Geometry check sheet. Reference: the model listing, model coordinates, mm. A direction names the side the tool comes from. Give positions to 0.01 mm unless a question says otherwise; leave off trailing zeros. Order: outer loops, then holes, each group sorted by start corner. A loop starts at its lowest first (then second) coordinate and runs counter-clockwise, first axis right, second up. Notation, with made-up numbers: (64.25, 38) - (114.25, 38) arc R27 cw to (114.25, 73) - close; hole circle Ø5 at (-28.75, 57.5). An arc over 180 degrees is marked (long way). Put each result on its own line as item: value. Start each with the question number.
```python
from build123d import *

# Parameters (mm, degrees)
CROQUIS3_W     = 1.65
CROQUIS3_H     = 8.851
MATRIZC1_COUNT = 2
MATRIZC1_ANGLE = 90


with BuildPart() as part:
    # Croquis1 → Revolución1 (revolve)
    with BuildSketch(Plane.XY):
        Polygon((8.85, 6.45), (8.85, 0), (2.5, 0), (2.5, 20.75), (8.85, 20.75), (8.85, 19.35), (6, 19.35), (6, 6.45), align=None)
    revolve(axis=Axis((0, 0, 0), (0, 1, 0)))

    # Croquis3 → Taladro roscado M41 (revolve, cut)
    with BuildSketch(Plane(origin=(0, 3.225, 0), x_dir=(0, 1, 0), z_dir=(1, 0, 0))):
        with Locations((0.825, 4.4255)):
            Rectangle(CROQUIS3_W, CROQUIS3_H)
    taladro_roscado_m41 = revolve(axis=Axis((0, 3.225, -6.35), (0, 0, 1)), mode=Mode.SUBTRACT)

    # MatrizC1: Taladro roscado M41 ×2 about axis
    matrizc1_axis = Axis((0, 0, 0), (0, -1, 0))
    for i in range(1, MATRIZC1_COUNT):
        add(taladro_roscado_m41.rotate(matrizc1_axis, i * MATRIZC1_ANGLE / (MATRIZC1_COUNT - 1)), mode=Mode.SUBTRACT)


solid = part.part
```
Item 1: Cross-section at A-A (z = 0). Enter the section's corners in (x, y) (3 decimals).
Item 2: Release check for a two-part mould opening along Y. For faces 1 (the face through (-0.073, 1.577, 5.415)), 2 (the face through (8.44, 20.04, -2.66)), 3 (the face through (2, 0, 2)), 4 (the face through (6, 19.35, 2)) record: +Y half, -Y half, draft (parallel to the pull), parting line (faces both ways), or undercut.
Item 3: Cross-section at C-C (z = 7.75). Enter the section's corners in (x, y) (3 decimals).
Item 4: Thickness scan on line 1 along Z through (x, y) = (0, 10.5); line 2 along Y through (x, z) = (-5.5, 5.75). Record the ranges inside material, lowest first.
Item 5: Cross-section at B-B (x = -7.5). Enter the section's corners in (y, z) (3 decimals), and give its area (3 significant figures).
Item 6: Cross-section at D-D (y = 2). Enter the section's corners in (x, z), and give its area (3 significant figures).
Item 7: Set-up check for faces 5 (the face through (8.44, 3.18, -2.66)), 6 (the face through (-5.413, 1.577, -0.073)), 7 (the face through (-6, 13, 0)): record each of +Z, -Z, +X, -X, +Y, -Y from which the full face is reachable in a straight line by a thin tool's end or side.
Item 8: Gauge pin test, flat ends, axial feed: pin 1 Ø10 at (y, z) = (14.5, 3) entering from -X; pin 2 Ø1.5 at (y, z) = (13, -2.5) entering from +X; pin 3 Ø2.5 at (y, z) = (3.225, 0) entering from -X; pin 4 Ø9 at (x, z) = (-2.5, -2.5) entering from -Y. Record the tip position at first contact, or that the pin passes through.
Recorded:
1. outline: (-8.85, 0) - (-2.5, 0) - (-2.5, 1.575) - (-8.85, 1.575) - close; (-8.85, 4.875) - (-2.5, 4.875) - (-2.5, 20.75) - (-8.85, 20.75) - (-8.85, 19.35) - (-6, 19.35) - (-6, 6.45) - (-8.85, 6.45) - close; (2.5, 0) - (8.85, 0) - (8.85, 6.45) - (6, 6.45) - (6, 19.35) - (8.85, 19.35) - (8.85, 20.75) - (2.5, 20.75) - close
2. face 1: undercut
2. face 2: draft
2. face 3: -Y half
2. face 4: undercut
3. outline: (-4.273, 0) - (4.273, 0) - (4.273, 6.45) - (-4.273, 6.45) - close; (-4.273, 19.35) - (4.273, 19.35) - (4.273, 20.75) - (-4.273, 20.75) - close; hole circle Ø3.3 at (0, 3.225)
4. line 1: z = -6 to -2.5, 2.5 to 6
4. line 2: y = 0 to 6.45, 19.35 to 20.75
5. outline: (0, -4.698) - (6.45, -4.698) - (6.45, 4.698) - (0, 4.698) - close; (19.35, -4.698) - (20.75, -4.698) - (20.75, 4.698) - (19.35, 4.698) - close; hole circle Ø3.3 at (3.225, 0)
5. area: 65.2 mm^2
6. outline: (-8.78, -1.11) arc R8.85 ccw (long way) to (1.11, 8.78) - (1.11, 2.24) arc R2.5 cw (long way) to (-2.24, -1.11) - close; (-8.78, 1.11) - (-2.24, 1.11) arc R2.5 cw to (-1.11, 2.24) - (-1.11, 8.78) arc R8.85 ccw to start
6. area: 198 mm^2
7. face 5: +Y, -Y
7. face 6: -X
7. face 7: none
8. pin 1: stops at x = -8.67
8. pin 2: stops at x = 5.74
8. pin 3: stops at x = 2.17
8. pin 4: stops at y = 0
